Design review of the part shown in the three views and the two pictorial views. Dimensions are in mm from the part's minimum x, y and z. A direction names the side the tool comes from. Give positions to 0.01 mm unless a question says otherwise; leave off trailing zeros. Loops run counter-clockwise (first coordinate to the right, second up) from the corner with the lowest first, then second, coordinate; pieces in that order, holes last.
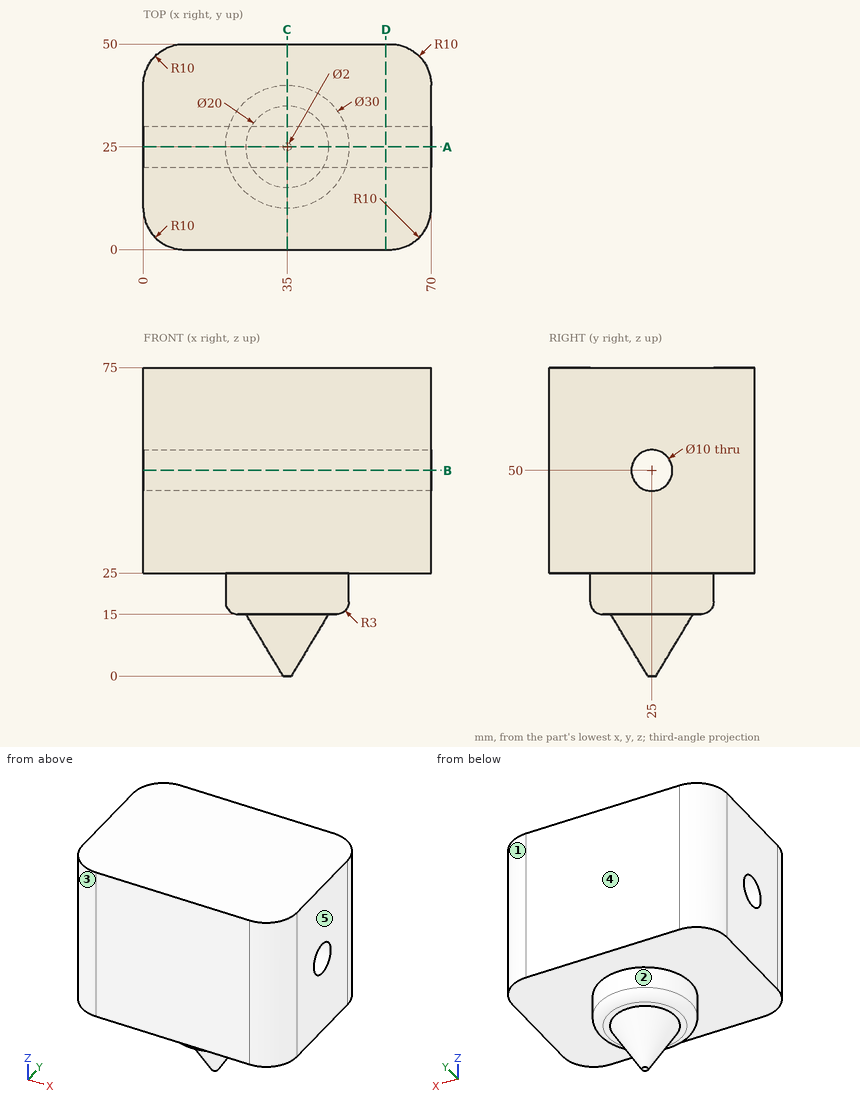
Q1. Take a section at A-A (y = 25). Give the boundary of the cut face in (x, z), plus the area to 3 significant figures.
Results:
outline: (0, 25) - (20, 25) - (20, 18) arc R3 ccw to (23, 15) - (25, 15) - (34, 0) - (36, 0) - (45, 15) - (47, 15) arc R3 ccw to (50, 18) - (50, 25) - (70, 25) - (70, 45) - (0, 45) - close; (0, 55) - (70, 55) - (70, 75) - (0, 75) - close
area: 3,260 mm2
Q2. Draft analysis for pull direction Y (two halves, no side actions). For the marked faces 3, 4 and 5, state which applies: pulls with the +Y half, pulls with the -Y half, needs draft (parallel to the pull), parting line crosses it, or undercut.
Results:
face 3: pulls with the -Y half
face 4: pulls with the +Y half
face 5: needs draft
Q3. Take a section at B-B (z = 50). Give the boundary of the cut face in (x, y), plus the area to 3 significant figures.
Results:
outline: (0, 10) arc R10 ccw to (10, 0) - (60, 0) arc R10 ccw to (70, 10) - (70, 20) - (0, 20) - close; (0, 30) - (70, 30) - (70, 40) arc R10 ccw to (60, 50) - (10, 50) arc R10 ccw to (0, 40) - close
area: 2,710 mm2
Q4. Take a section at C-C (x = 35). Give the boundary of the cut face in (y, z), plus the area to 3 significant figures.
Results:
outline: (0, 25) - (10, 25) - (10, 18) arc R3 ccw to (13, 15) - (15, 15) - (24, 0) - (26, 0) - (35, 15) - (37, 15) arc R3 ccw to (40, 18) - (40, 25) - (50, 25) - (50, 75) - (0, 75) - close; hole circle Ø10 at (25, 50)
area: 2,880 mm2
Q5. Wall thickness on line 1 (Y direction, x = 50, z = 50); line 2 (Z direction, x = 3, y = 37); line 3 (X direction, y = 36.5, z = 22): over which ranges is each line inside the solid? List them lowest first.
Results:
line 1: y = 0 to 20, 30 to 50
line 2: z = 25 to 75
line 3: x = 25.37 to 44.63
Q6. Tool access review of the marked faces 1 and 2: name each direction out of +Z, -Z, +X, -X, +Y, -Y from which nothing blocks a thin tool from reaching the whole face with its end or side.
Results:
face 1: +Z, -Z, +X, +Y
face 2: -Z
Q7. Insertion check: pin 1 (1.5 mm diameter, centred on x = 55.5, y = 44, fed in from -Z); pin 2 (6 mm diameter, centred on y = 6.5, z = 36, fed in from +X); pin 3 (8 mm diameter, centred on x = 50, z = 16.5, fed in from -Y). Each pin has a flat end and moves straight along its axis. Give the tip position at first contact, or say it passes through.
Results:
pin 1: stops at z = 25
pin 2: stops at x = 69.99
pin 3: stops at y = 15
Q8. Take a section at D-D (x = 59). Give the boundary of the cut face in (y, z).
Results:
outline: (0, 25) - (50, 25) - (50, 75) - (0, 75) - close; hole circle Ø10 at (25, 50)
